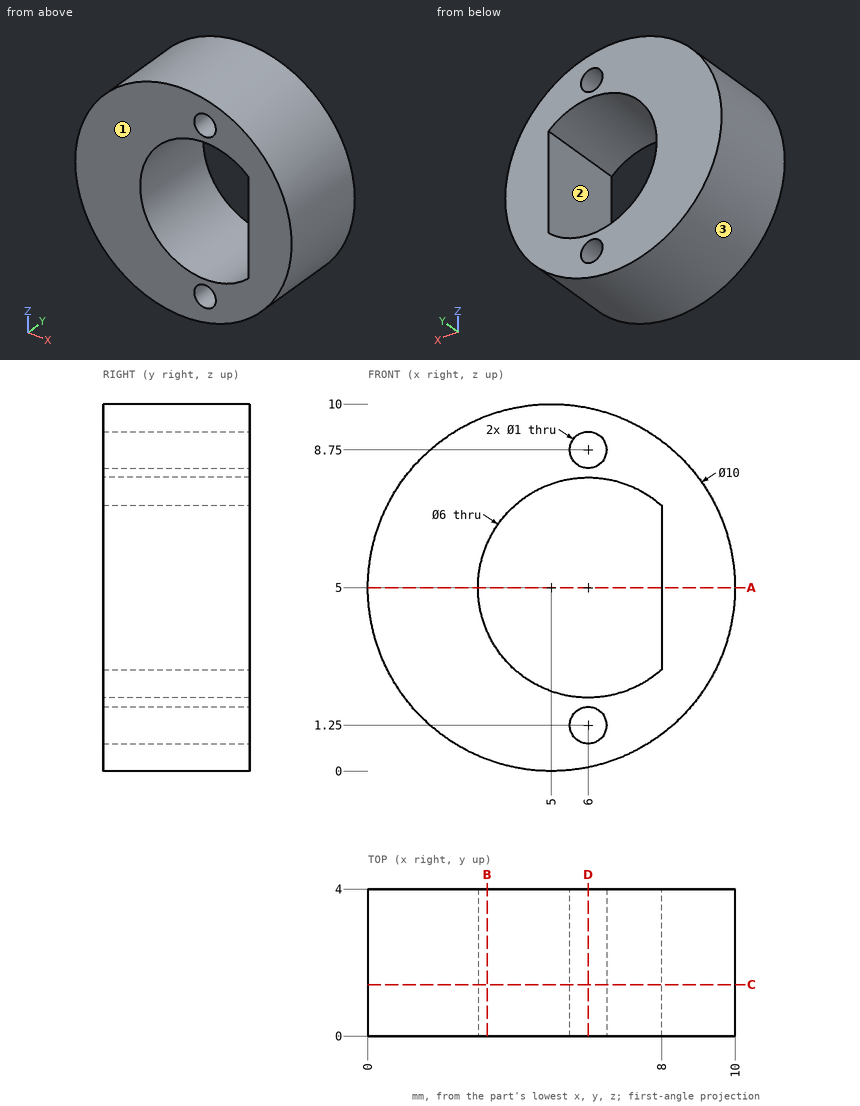
Print and shaded views of the part. All mm, measured from the part's lowest x, y and z. Give positions to 0.01 mm unless a question says otherwise; leave off trailing zeros. Order: outer loops, then holes, each group sorted by start corner. A loop starts at its lowest first (then second) coordinate and runs counter-clockwise, first axis right, second up. Notation, with made-up numbers: (43.25, 51) - (94.25, 51) arc R25 cw to (94.25, 71) - close; hole circle Ø7 at (74.5, 23). An arc over 180 degrees is marked (long way). Use a Markdown table: item, result.
1) Two-plate mould, pull along Z, no slides. Class the marked faces 1, 2 and 3: +Z half, -Z half, draft (parallel to the pull), parting line (faces both ways), or undercut.
Checked values:
| item | result |
|---|---|
| face 1 | draft |
| face 2 | undercut |
| face 3 | parting line |
2) Flat gauge pins, fed straight in: P1, Ø1, axis at x = 7.5, y = 1.5, coming from the +Z side; P2, Ø2, axis at x = 7.5, z = 5.5, coming from the -Y side; P3, Ø1, axis at y = 3, z = 3, coming from the +X side; P4, Ø3.5, axis at x = 6, z = 5, coming from the -Y side. Where does each tip first touch, or does it go through?
Checked values:
| item | result |
|---|---|
| P1 | z = 9.58 |
| P2 | y = 0 |
| P3 | x = 9.77 |
| P4 | through |
3) Saw through at B-B on x = 3.25. List the corners of the cut face in (y, z).
Checked values:
| item | result |
|---|---|
| outline | (0, 0.32) - (4, 0.32) - (4, 3.8) - (0, 3.8) - close; (0, 6.2) - (4, 6.2) - (4, 9.68) - (0, 9.68) - close |
4) Saw through at C-C on y = 1.4. List the corners of the cut face in (x, z), plus the area to 3 significant figures.
Checked values:
| item | result |
|---|---|
| outline | circle Ø10 at (5, 5); hole circle Ø1 at (6, 1.25); hole circle Ø1 at (6, 8.75); hole (8, 2.76) - (8, 7.24) arc R3 ccw (long way) to start |
| area | 51.8 mm² |
5) Saw through at D-D on x = 6. List the corners of the cut face in (y, z), plus the area to 3 significant figures.
Checked values:
| item | result |
|---|---|
| outline | (0, 0.1) - (4, 0.1) - (4, 0.75) - (0, 0.75) - close; (0, 1.75) - (4, 1.75) - (4, 2) - (0, 2) - close; (0, 8) - (4, 8) - (4, 8.25) - (0, 8.25) - close; (0, 9.25) - (4, 9.25) - (4, 9.9) - (0, 9.9) - close |
| area | 7.19 mm² |
6) Probe L1, parallel to Z at x = 6, y = 1.4; L2, parallel to Z at x = 4.5, y = 0.4; L3, parallel to X at y = 0.55, z = 3. List the from-to ranges inside material, lowest first. Write a range as from..to.
Checked values:
| item | result |
|---|---|
| L1 | 0.1..0.75, 1.75..2, 8..8.25, 9.25..9.9 |
| L2 | 0.03..2.4, 7.6..9.97 |
| L3 | 0.42..3.76, 8..9.58 |
7) Saw through at A-A on z = 5. List the corners of the cut face in (x, y), plus the area to 3 significant figures.
Checked values:
| item | result |
|---|---|
| outline | (0, 0) - (3, 0) - (3, 4) - (0, 4) - close; (8, 0) - (10, 0) - (10, 4) - (8, 4) - close |
| area | 20.0 mm² |
